Verification items for the finished model (mm, model axes). A direction names the side the tool comes from. Give positions to 0.01 mm unless a question says otherwise; leave off trailing zeros. Write each loop counter-clockwise with the first axis right and the second up, starting at its lowest first coordinate (ties: lowest second). Pieces come first, ordered by that corner, then holes.
from build123d import *

# Parameters (mm, degrees)
BOX044_W                                   = 19
BOX044_H                                   = 29
BOX044_DEPTH                               = 14
BOX043_W                                   = 23
BOX043_H                                   = 10
BOX043_DEPTH                               = 14
CYLINDER012_R                              = 1.9
CYLINDER012_DEPTH                          = 10
CYLINDER014_R                              = 3.5
CYLINDER014_DEPTH                          = 2
CYLINDER013_R                              = 1.65
CYLINDER013_DEPTH                          = 10
CYLINDER010_R                              = 1.6
CYLINDER010_DEPTH                          = 18
CYLINDER011_R                              = 1.9
CYLINDER011_DEPTH                          = 18
BOX015_W                                   = 5.75
BOX015_H                                   = 13
BOX015_DEPTH                               = 25
CHAMFER016016006_SIZE                      = 0.4
BOX009_W                                   = 16
BOX009_H                                   = 24
BOX009_DEPTH                               = 4.5
FILLET001_R                                = 7
CHAMFER011_SIZE                            = 5
BOX010_W                                   = 16
BOX010_H                                   = 24
BOX010_DEPTH                               = 6.5
FILLET002_R                                = 7
CHAMFER009_SIZE                            = 5
BOX012_W                                   = 43.5
BOX012_H                                   = 8
BOX012_DEPTH                               = 25
BOX008_W                                   = 52
BOX008_H                                   = 8
BOX008_DEPTH                               = 25
CHAMFER016016004_SIZE                      = 5
BOX011_W                                   = 21.75
BOX011_H                                   = 13
BOX011_DEPTH                               = 14
CHAMFER016016005_SIZE                      = 5
CHAMFER016016007_SIZE                      = 0.4
CHAMFER016016008004017002013005003_SIZE    = 1
CHAMFER016016008004017002013005004_SIZE    = 1
CHAMFER016016008004017002013005004002_SIZE = 0.4


with BuildPart() as cube044:
    # Box044 → Box044 (new body)
    with BuildSketch(Plane(origin=(5, -40.5, -20.5), x_dir=(1, 0, 0), z_dir=(0, 0, 1))):
        with Locations((9.5, 14.5)):
            Rectangle(BOX044_W, BOX044_H)
    extrude(amount=BOX044_DEPTH)


with BuildPart() as cube043:
    # Box043 → Box043 (new body)
    with BuildSketch(Plane(origin=(0, -29, -20.5), x_dir=(1, 0, 0), z_dir=(0, 0, 1))):
        with Locations((11.5, 5)):
            Rectangle(BOX043_W, BOX043_H)
    extrude(amount=BOX043_DEPTH)


with BuildPart() as cylinder012:
    # Cylinder012 → Cylinder012 (new body)
    with BuildSketch(Plane(origin=(-15, -37.5, -12.5), x_dir=(1, 0, 0), z_dir=(0, 1, 0))):
        Circle(CYLINDER012_R)
    extrude(amount=CYLINDER012_DEPTH)


with BuildPart() as cylinder014:
    # Cylinder014 → Cylinder014 (new body)
    with BuildSketch(Plane(origin=(-37.5, -39, -12.5), x_dir=(1, 0, 0), z_dir=(0, 1, 0))):
        Circle(CYLINDER014_R)
    extrude(amount=CYLINDER014_DEPTH)


with BuildPart() as fusion011:
    # Cylinder013 → Cylinder013 (new body)
    with BuildSketch(Plane(origin=(-37.5, -41.5, -12.5), x_dir=(1, 0, 0), z_dir=(0, 1, 0))):
        Circle(CYLINDER013_R)
    extrude(amount=CYLINDER013_DEPTH)

    # Fusion011: union Cylinder012, Cylinder014
    add(cylinder012.part)
    add(cylinder014.part)


with BuildPart() as cylinder010:
    # Cylinder010 → Cylinder010 (new body)
    with BuildSketch(Plane(origin=(10, -20, -30), x_dir=(1, 0, 0), z_dir=(0, 0, 1))):
        Circle(CYLINDER010_R)
    extrude(amount=CYLINDER010_DEPTH)


with BuildPart() as fusion010:
    # Cylinder011 → Cylinder011 (new body)
    with BuildSketch(Plane(origin=(10, -20, -11), x_dir=(1, 0, 0), z_dir=(0, 0, 1))):
        Circle(CYLINDER011_R)
    extrude(amount=CYLINDER011_DEPTH)

    # Fusion010: union Cylinder010
    add(cylinder010.part)


with BuildPart() as fusion010_1:
    # Fusion010 placement: moved
    add(fusion010.part.moved(Location((4, 0, 0))))


with BuildPart() as chamfer016016006:
    # Box015 → Box015 (new body)
    with BuildSketch(Plane(origin=(0.25, -39, -25), x_dir=(1, 0, 0), z_dir=(0, 0, 1))):
        with Locations((2.875, 6.5)):
            Rectangle(BOX015_W, BOX015_H)
    extrude(amount=BOX015_DEPTH)

    # Chamfer016016006
    chamfer016016006_edges = [chamfer016016006.edges().sort_by_distance(p)[0] for p in [
        (0.25, -26, -12.5),
    ]]
    chamfer(chamfer016016006_edges, length=CHAMFER016016006_SIZE)


with BuildPart() as chamfer011:
    # Box009 → Box009 (new body)
    with BuildSketch(Plane(origin=(2, -39, -25), x_dir=(1, 0, 0), z_dir=(0, 0, 1))):
        with Locations((8, 12)):
            Rectangle(BOX009_W, BOX009_H)
    extrude(amount=BOX009_DEPTH)

    # Fillet001
    fillet001_edges = [chamfer011.edges().sort_by_distance(p)[0] for p in [
        (2, -15, -22.75),
        (18, -15, -22.75),
    ]]
    fillet(fillet001_edges, radius=FILLET001_R)

    # Chamfer011
    chamfer011_edges = [chamfer011.edges().sort_by_distance(p)[0] for p in [
        (18, -39, -22.75),
    ]]
    chamfer(chamfer011_edges, length=CHAMFER011_SIZE)


with BuildPart() as chamfer011_1:
    # Chamfer011 placement: moved
    add(chamfer011.part.moved(Location((4, 0, 0))))


with BuildPart() as chamfer009:
    # Box010 → Box010 (new body)
    with BuildSketch(Plane(origin=(2, -39, -6.5), x_dir=(1, 0, 0), z_dir=(0, 0, 1))):
        with Locations((8, 12)):
            Rectangle(BOX010_W, BOX010_H)
    extrude(amount=BOX010_DEPTH)

    # Fillet002
    fillet002_edges = [chamfer009.edges().sort_by_distance(p)[0] for p in [
        (2, -15, -3.25),
        (18, -15, -3.25),
    ]]
    fillet(fillet002_edges, radius=FILLET002_R)

    # Chamfer009
    chamfer009_edges = [chamfer009.edges().sort_by_distance(p)[0] for p in [
        (18, -39, -3.25),
    ]]
    chamfer(chamfer009_edges, length=CHAMFER009_SIZE)


with BuildPart() as chamfer009_1:
    # Chamfer009 placement: moved
    add(chamfer009.part.moved(Location((4, 0, 0))))


with BuildPart() as cube012:
    # Box012 → Box012 (new body)
    with BuildSketch(Plane(origin=(-48, -34, -25), x_dir=(1, 0, 0), z_dir=(0, 0, 1))):
        with Locations((21.75, 4)):
            Rectangle(BOX012_W, BOX012_H)
    extrude(amount=BOX012_DEPTH)


with BuildPart() as chamfer016016004:
    # Box008 → Box008 (new body)
    with BuildSketch(Plane(origin=(-45, -39, -25), x_dir=(1, 0, 0), z_dir=(0, 0, 1))):
        with Locations((26, 4)):
            Rectangle(BOX008_W, BOX008_H)
    extrude(amount=BOX008_DEPTH)

    # Cut010011006: cut Cube012
    add(cube012.part, mode=Mode.SUBTRACT)

    # Chamfer016016004
    chamfer016016004_edges = [chamfer016016004.edges().sort_by_distance(p)[0] for p in [
        (-45, -36.5, 0),
        (-45, -36.5, -25),
    ]]
    chamfer(chamfer016016004_edges, length=CHAMFER016016004_SIZE)


with BuildPart() as chamfer016016008004017002013005004002:
    # Box011 → Box011 (new body)
    with BuildSketch(Plane(origin=(0.25, -39, -20.5), x_dir=(1, 0, 0), z_dir=(0, 0, 1))):
        with Locations((10.875, 6.5)):
            Rectangle(BOX011_W, BOX011_H)
    extrude(amount=BOX011_DEPTH)

    # Chamfer016016005
    chamfer016016005_edges = [chamfer016016008004017002013005004002.edges().sort_by_distance(p)[0] for p in [
        (22, -39, -13.5),
    ]]
    chamfer(chamfer016016005_edges, length=CHAMFER016016005_SIZE)

    # Chamfer016016007
    chamfer016016007_edges = [chamfer016016008004017002013005004002.edges().sort_by_distance(p)[0] for p in [
        (0.25, -26, -13.5),
    ]]
    chamfer(chamfer016016007_edges, length=CHAMFER016016007_SIZE)

    # Fusion017: union Chamfer016016006, Chamfer011, Chamfer009, Chamfer016016004
    add(chamfer016016006.part)
    add(chamfer011_1.part)
    add(chamfer009_1.part)
    add(chamfer016016004.part)

    # Cut010011007: cut Fusion010
    add(fusion010_1.part, mode=Mode.SUBTRACT)

    # Cut010011008: cut Fusion011
    add(fusion011.part, mode=Mode.SUBTRACT)

    # Cut010011008009003016026002: cut Cube043
    add(cube043.part, mode=Mode.SUBTRACT)

    # Chamfer016016008004017002013005003
    chamfer016016008004017002013005003_edges = [chamfer016016008004017002013005004002.edges().sort_by_distance(p)[0] for p in [
        (22, -29, -13.5),
        (0.25, -29, -13.5),
    ]]
    chamfer(chamfer016016008004017002013005003_edges, length=CHAMFER016016008004017002013005003_SIZE)

    # Cut010011008009003016026003: cut Cube044
    add(cube044.part, mode=Mode.SUBTRACT)

    # Chamfer016016008004017002013005004
    chamfer016016008004017002013005004_edges = [chamfer016016008004017002013005004002.edges().sort_by_distance(p)[0] for p in [
        (5, -39, -13.5),
    ]]
    chamfer(chamfer016016008004017002013005004_edges, length=CHAMFER016016008004017002013005004_SIZE)

    # Chamfer016016008004017002013005004002
    chamfer016016008004017002013005004002_edges = [chamfer016016008004017002013005004002.edges().sort_by_distance(p)[0] for p in [
        (3.325, -26, -25),
        (0.45, -26.2, -25),
        (6, -24, -25),
        (8.050253, -17.050253, -25),
        (14, -15, -25),
        (22, -28, -25),
        (19.5, -36.5, -25),
        (19.949747, -17.050253, -25),
        (-11.5, -39, 0),
        (-42.5, -39, -2.5),
        (-45, -39, -12.5),
        (-42.5, -39, -22.5),
        (-11.5, -39, -25),
        (3.325, -26, 0),
        (0.45, -26.2, 0),
        (6, -24, 0),
        (8.050253, -17.050253, 0),
        (14, -15, 0),
        (22, -28, 0),
        (19.5, -36.5, 0),
        (19.949747, -17.050253, 0),
        (-2.125, -31, -25),
        (-2.125, -31, 0),
        (-4.5, -32.5, 0),
        (-4.5, -32.5, -25),
        (-42.5, -34, -22.5),
        (-45, -34, -12.5),
        (-42.5, -34, -2.5),
        (-22.25, -34, -25),
        (-22.25, -34, 0),
        (0.25, -28.7, -25),
        (0.25, -28.7, 0),
    ]]
    chamfer(chamfer016016008004017002013005004002_edges, length=CHAMFER016016008004017002013005004002_SIZE)


with BuildPart() as part_mirroring002:
    # Part__Mirroring002: instance of Chamfer016016008004017002013005004002
    add(chamfer016016008004017002013005004002.part.mirror(Plane(origin=(0, 0, 0), x_dir=(0, 1, 0), z_dir=(0, 0, 1))))


solid = part_mirroring002.part
Item 1: Sectioned sample at C-C on x = -28. Record the cut outline in (y, z), then the cut area to 3 significant figures.
Answer key:
outline: (-39, 0.4) - (-38.6, 0) - (-34.4, 0) - (-34, 0.4) - (-34, 24.6) - (-34.4, 25) - (-38.6, 25) - (-39, 24.6) - close
area: 125 mm2
Item 2: Set-up check for faces 1 (the face through (6, -24, 23)), 2 (the face through (8.2, -17.31, 0.11)): record each of +Z, -Z, +X, -X, +Y, -Y from which the full face is reachable in a straight line by a thin tool's end or side.
Answer key:
face 1: +Z, -Z, -X, +Y
face 2: -Z, -X, +Y
Item 3: Scan lines: line 1 along Z through (x, y) = (8, -30); line 2 along Y through (x, z) = (14, 23.9); line 3 along Y through (x, z) = (14, 5). Record each from-to range of solid material in increasing order.
Answer key:
line 1: z = 0 to 6.5, 20.5 to 25
line 2: y = -39 to -21.6, -18.4 to -15
line 3: y = -39 to -21.9, -18.1 to -15
Item 4: Sectioned sample at D-D on x = 14. Record the cut outline in (y, z).
Answer key:
outline: (-39, 0.4) - (-38.6, 0) - (-21.9, 0) - (-21.9, 6.5) - (-39, 6.5) - close; (-39, 20.5) - (-21.6, 20.5) - (-21.6, 25) - (-38.6, 25) - (-39, 24.6) - close; (-18.4, 20.5) - (-15, 20.5) - (-15, 24.6) - (-15.4, 25) - (-18.4, 25) - close; (-18.1, 0) - (-15.4, 0) - (-15, 0.4) - (-15, 6.5) - (-18.1, 6.5) - close
Item 5: Sectioned sample at B-B on x = -37.5. Record the cut outline in (y, z).
Answer key:
outline: (-39, 0.4) - (-38.6, 0) - (-34.4, 0) - (-34, 0.4) - (-34, 10.85) - (-37, 10.85) - (-37, 9) - (-39, 9) - close; (-39, 16) - (-37, 16) - (-37, 14.15) - (-34, 14.15) - (-34, 24.6) - (-34.4, 25) - (-38.6, 25) - (-39, 24.6) - close
Item 6: Depth check by flat-ended pin: pin 1 (1.5 mm diameter, centred on y = -32.5, z = 10, fed in from -X); pin 2 (1 mm diameter, centred on x = 1, z = 3.5, fed in from +Y); pin 3 (2.5 mm diameter, centred on x = -3, z = 6.5, fed in from +Y); pin 4 (2.5 mm diameter, centred on x = -37.5, z = 12.5, fed in from -Y). Enter the tip coordinate at first touch or a pass-through.
Answer key:
pin 1: stops at x = -4.5
pin 2: stops at y = -26
pin 3: stops at y = -31
pin 4: passes through
Item 7: Sectioned sample at A-A on z = 12.5. Record the cut outline in (x, y), then the cut area to 3 significant figures.
Answer key:
outline: (-45, -38.6) - (-44.6, -39) - (-41, -39) - (-41, -37) - (-39.15, -37) - (-39.15, -34) - (-44.6, -34) - (-45, -34.4) - close; (-35.85, -37) - (-34, -37) - (-34, -39) - (4, -39) - (5, -38) - (5, -29) - (1.25, -29) - (0.25, -30) - (0.25, -31) - (-4.5, -31) - (-4.5, -34) - (-13.1, -34) - (-13.1, -37.5) - (-16.9, -37.5) - (-16.9, -34) - (-35.85, -34) - close
area: 250 mm2
Item 8: Release check for a two-part mould opening along Z. For faces 3 (the face through (20, -36, 3)), 4 (the face through (19.326, -36.396, 0.203)), 5 (the face through (-42.392, -34.197, 22.322)), 6 (the face through (13, -27, 20.5)) record: released by +Z, released by -Z, zero draft, split by the parting line, or undercut.
Answer key:
face 3: zero draft
face 4: released by -Z
face 5: released by +Z
face 6: undercut
